Read the model definition and answer for the solid it produces. Units are mm, in the model's axes. Face numbers are marked on the shaded views. Coordinates: 2 decimals unless noted, no trailing zeros. Write each loop counter-clockwise with the first axis right and the second up, starting at its lowest first coordinate (ties: lowest second). Pieces come first, ordered by that corner, then holes. Notation, with made-up numbers: (28.25, 82.25) -> (43.25, 82.25) arc R19 cw to (43.25, 97.25) -> close; hole circle Ø8 at (76, 2). An arc over 180 degrees is marked (long way). One line per item, written item: value. Start each with the question number.
1. For a pull along X with two mould halves and no side action, classify the marked faces 1, 2 and 3 as pulls with the +X half, pulls with the -X half, needs draft (parallel to the pull), parting line crosses it, or undercut.
2. Find section A-A, the plane y = -16. Write down the section's boundary in (x, z), and give its area (3 significant figures).
3. Find section D-D, the plane y = -35. Write down the section's boundary in (x, z), and give its area (3 significant figures).
4. Find section B-B, the plane x = 0. Write down the section's boundary in (y, z).
5. Consider line 1 along X through (y, z) = (-22.5, -3); line 2 along Y through (x, z) = (43.5, 16.5); line 3 along X through (y, z) = (-27, -6.5). Determine where each line is inside the solid, lowest interval first.
6. Given P1, Ø2, axis at y = -8.5, z = -10.5, coming from the -X side; P2, Ø4, axis at y = -30.5, z = 19, coming from the +X side; P3, Ø4, axis at x = 54.5, z = 20.5, coming from the +Y side; P4, Ø1, axis at y = -43, z = -1.5, coming from the +X side, each flat-ended and moving along its own axis, determine where each tip first touches the part or whether it passes through.
7. Find section C-C, the plane z = 7. State how many separate pieces and enclosed holes the cut face has, and give its area (3 significant figures).
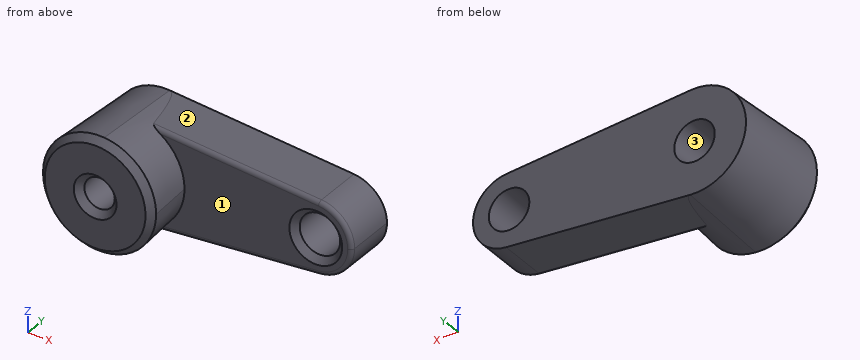
```python
from build123d import *

# Parameters (mm, degrees)
F0_R     = 9.8233576781
F1_DEPTH = 25
F2_DEPTH = 50
F2_TAPER = -3
F4_R     = 2


# Not quite as in the source:
# - a fillet or chamfer that OpenCascade refuses, or shapes differently, is made with other operations: its cross-section is extruded or revolved along the edge and cut away or added


with BuildPart() as f1:
    # F0 (on Front) → F1 (new body)
    with BuildSketch(Plane.XZ):
        with BuildLine():
            ThreePointArc((2.0833333333, 24.9130432148), (18.3995018048, 16.9250800097), (25, 0))
            ThreePointArc((25, 0), (18.3995018048, -16.9250800097), (2.0833333333, -24.9130432148))
            Line((2.0833333333, -24.9130432148), (91.4583333333, -17.4391302504))
            ThreePointArc((91.4583333333, -17.4391302504), (72.5, 0), (91.4583333333, 17.4391302504))
            Line((91.4583333333, 17.4391302504), (2.0833333333, 24.9130432148))
        make_face()
        with BuildLine():
            ThreePointArc((2.0833333333, -24.9130432148), (18.3995018048, -16.9250800097), (25, 0))
            ThreePointArc((25, 0), (18.3995018048, 16.9250800097), (2.0833333333, 24.9130432148))
            ThreePointArc((2.0833333333, 24.9130432148), (-25, 0), (2.0833333333, -24.9130432148))
        make_face()
        Circle(F0_R, mode=Mode.SUBTRACT)
        with BuildLine():
            ThreePointArc((107.5, 0), (102.8796512634, 11.8475560068), (91.4583333333, 17.4391302504))
            ThreePointArc((91.4583333333, 17.4391302504), (72.5, 0), (91.4583333333, -17.4391302504))
            ThreePointArc((91.4583333333, -17.4391302504), (102.8796512634, -11.8475560068), (107.5, 0))
        make_face()
        with Locations((90, 0)):
            Circle(F0_R, mode=Mode.SUBTRACT)
    extrude(amount=F1_DEPTH)

    # F0 (on Front) → F2 (join)
    with BuildSketch(Plane.XZ):
        with BuildLine():
            ThreePointArc((2.0833333333, -24.9130432148), (18.3995018048, -16.9250800097), (25, 0))
            ThreePointArc((25, 0), (18.3995018048, 16.9250800097), (2.0833333333, 24.9130432148))
            ThreePointArc((2.0833333333, 24.9130432148), (-25, 0), (2.0833333333, -24.9130432148))
        make_face()
        Circle(F0_R, mode=Mode.SUBTRACT)
    extrude(amount=F2_DEPTH, taper=F2_TAPER)

    # F3: chamfer of 3 on 3 edges, made by hand

    # F3_s1 → F3_t2 (revolve, cut)
    with BuildSketch(Plane.XY):
        Polygon((102.8233576781, -25), (99.8233576781, -22), (99.8233576781, -25), align=None)
    revolve(axis=Axis((90, -25, 0), (0, -1, 0)), mode=Mode.SUBTRACT)

    # F3_s3 → F3_t4 (revolve, cut)
    with BuildSketch(Plane.XY):
        Polygon((7.3684204855, -46.8429921313), (10.3643090898, -50), (7.2029687139, -50), align=None)
    revolve(axis=Axis((0, -50, 0), (0, 1, 0)), mode=Mode.SUBTRACT)

    # F3_s5 → F3_t6 (revolve, cut)
    with BuildSketch(Plane(origin=(0, 0, 0), x_dir=(0, 1, 0), z_dir=(0.9965217286, 0, 0.0833333333))):
        Polygon((-46.8429921313, -27.4549371926), (-50, -24.4590485883), (-50, -27.6203889642), align=None)
    revolve(axis=Axis((0, -50, 0), (0, 1, 0)), mode=Mode.SUBTRACT)

    # F4
    f4_edges = [f1.edges().sort_by_distance(p)[0] for p in [
        (50.856157, -25, -20.834455),
        (107.5, -25, 0),
        (50.856157, -25, 20.834455),
    ]]
    fillet(f4_edges, radius=F4_R)


solid = f1.part
```
Answer block:
1. face 1: needs draft
1. face 2: pulls with the +X half
1. face 3: undercut
2. outline: (8.59, -24.37) -> (91.46, -17.44) arc R17.5 ccw to (91.46, 17.44) -> (8.59, 24.37) arc R25.84 ccw (long way) to start; hole circle Ø17.97 at (0, 0); hole circle Ø19.65 at (90, 0)
2. area: 4,820 mm2
3. outline: circle Ø53.67 at (0, 0); hole circle Ø15.98 at (0, 0)
3. area: 2,060 mm2
4. outline: (-50, -24.46) -> (-46.84, -27.45) -> (0, -25) -> (0, -9.82) -> (-46.84, -7.37) -> (-50, -10.36) -> close; (-50, 10.36) -> (-46.84, 7.37) -> (0, 9.82) -> (0, 25) -> (-46.84, 27.45) -> (-50, 24.46) -> close
5. line 1: x = -26.01 to -8.11, 8.11 to 80.12, 99.88 to 107.24
5. line 2: y = -25 to 0
5. line 3: x = -25.6 to -5.33, 5.33 to 25.6
6. P1: stops at x = -23.61
6. P2: stops at x = 20.46
6. P3: stops at y = 0
6. P4: stops at x = 27.25
7. separate pieces: 3
7. enclosed holes: 0
7. area: 3,710 mm2
